Input: part model. Units: mm. Frame: model coordinates. Face numbers are marked on the shaded views. A direction names the side the tool comes from. Give positions to 0.01 mm unless a question says otherwise; leave off trailing zeros. Write each loop counter-clockwise with the first axis right and the second up, starting at its lowest first coordinate (ties: lowest second). Pieces come first, ordered by that corner, then holes. Notation, with made-up numbers: (74.25, 33) -> (92.25, 33) arc R9 ccw to (92.25, 44) -> close; hole circle Ø3 at (-23.75, 1). An arc over 180 degrees is marked (long way). Return JSON: item names as keys, results as strings. Group by question number.
Item 1: Pin query (flat end, axial travel): P1, Ø6, axis at x = 9.5, y = -38.5, coming from the -Z side; P2, Ø16.5, axis at x = -8, y = 19.5, coming from the +Z side; P3, Ø12, axis at y = -36.5, z = 13, coming from the -X side; P4, Ø2, axis at y = 17.5, z = 13.5, coming from the +X side. Return the tip coordinate at first contact, or that it passes through.
Item 2: Section D-D, the plane y = 48. Return loops of the section in (x, z), then the cut area to 3 significant figures.
Item 3: Line query: line 1 (X direction, y = -46, z = 23); line 2 (X direction, y = 7, z = 27.5); line 3 (Y direction, x = 11, z = 9.5). Output: solid intervals per line, ascending. Write a range as [from, to].
Item 4: Section B-B, the plane x = 11. Return loops of the section in (y, z), then the cut area to 3 significant figures.
Item 5: Section C-C, the plane y = 5.5. Return loops of the section in (x, z).
Item 6: Mould query, pull axis Y, two halves, no side actions, for the marked faces 1, 2 and 3. Classes: released by +Y, released by -Y, zero draft, split by the parting line, or undercut.
Item 7: Set-up query: the marked faces 4 and 5. Return all of +Z, -Z, +X, -X, +Y, -Y with unobstructed straight access to the full face (end or side cutting, diameter ignored); none if empty.
Item 8: Section A-A, the plane z = 29. Return loops of the section in (x, y).
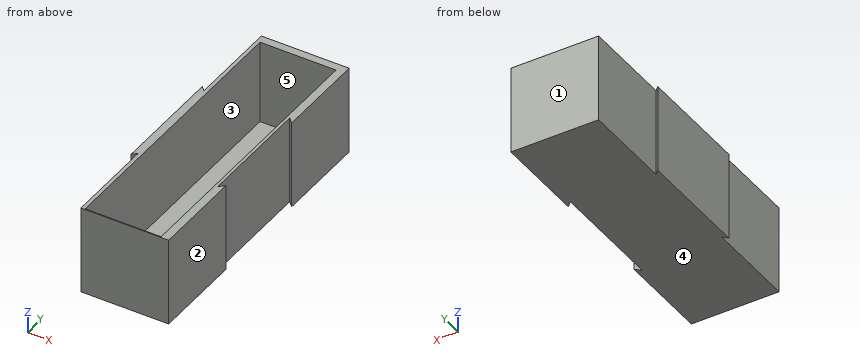
from build123d import *

# Parameters (mm, degrees)
F0_W     = 39.7
F0_H     = 125.2
F0_W_2   = 32.7
F0_H_2   = 118.2
F1_DEPTH = 2
F2_DEPTH = 38
F4_DEPTH = 38.001
F5_SIZE  = 3.1


with BuildPart() as f1:
    # F0 (on Top) → F1 (new body)
    with BuildSketch(Plane.XY):
        Rectangle(F0_W, F0_H)
        Rectangle(F0_W_2, F0_H_2, mode=Mode.SUBTRACT)
        Rectangle(F0_W_2, F0_H_2)
    extrude(amount=F1_DEPTH)

    # F0 (on Top) → F2 (join)
    with BuildSketch(Plane.XY):
        Rectangle(F0_W, F0_H)
        Rectangle(F0_W_2, F0_H_2, mode=Mode.SUBTRACT)
    extrude(amount=F2_DEPTH)

    # F3 (on face) → F4 (cut, through all)
    with BuildSketch(Plane.XY.offset(38)):
        Polygon((-17.953553, 22.75), (-17.953553, 62.6), (-19.85, 62.6), (-19.85, 24.646447), align=None)
        Polygon((-19.85, -62.6), (-17.953553, -62.6), (-17.953553, -22.75), (-19.85, -24.646447), align=None)
        Polygon((19.85, -22.75), (19.85, 22.75), (17.6, 25), (17.6, -25), align=None)
    extrude(amount=-F4_DEPTH, mode=Mode.SUBTRACT)

    # F5
    f5_edges = [f1.edges().sort_by_distance(p)[0] for p in [
        (0, -59.1, 38),
    ]]
    chamfer(f5_edges, length=F5_SIZE)


solid = f1.part
Answer below:
{
 "1": {"P1": "stops at z = 0", "P2": "stops at z = 2", "P3": "stops at x = -17.95", "P4": "stops at x = 17.6"},
 "2": {"outline": "(-17.95, 0) -> (19.85, 0) -> (19.85, 38) -> (16.35, 38) -> (16.35, 2) -> (-16.35, 2) -> (-16.35, 38) -> (-17.95, 38) -> close", "area": "259 mm2"},
 "3": {"line 1": "x = [-17.95, -16.35], [16.35, 19.85]", "line 2": "x = [-19.85, -16.35], [16.35, 17.6]", "line 3": "y = [-62.6, -59.1], [59.1, 62.6]"},
 "4": {"outline": "(-62.6, 0) -> (62.6, 0) -> (62.6, 38) -> (59.1, 38) -> (59.1, 2) -> (-59.1, 2) -> (-59.1, 34.9) -> (-62.2, 38) -> (-62.6, 38) -> close", "area": "498 mm2"},
 "5": {"outline": "(-19.85, 0) -> (17.6, 0) -> (17.6, 38) -> (16.35, 38) -> (16.35, 2) -> (-16.35, 2) -> (-16.35, 38) -> (-19.85, 38) -> close"},
 "6": {"face 1": "released by +Y", "face 2": "zero draft", "face 3": "undercut"},
 "7": {"face 4": "-Z, +X, -X, +Y, -Y", "face 5": "+Z"},
 "8": {"outline": "(-19.85, -24.65) -> (-17.95, -22.75) -> (-17.95, -62.6) -> (19.85, -62.6) -> (19.85, -22.75) -> (17.6, -25) -> (17.6, 25) -> (19.85, 22.75) -> (19.85, 62.6) -> (-17.95, 62.6) -> (-17.95, 22.75) -> (-19.85, 24.65) -> close; hole (-16.35, -59.1) -> (16.35, -59.1) -> (16.35, 59.1) -> (-16.35, 59.1) -> close"}
}
